Read the model definition and answer for the solid it produces. Units are mm, in the model's axes. A direction names the side the tool comes from. Give positions to 0.01 mm unless a question says otherwise; leave off trailing zeros. Order: outer loops, then holes, each group sorted by start corner. A loop starts at its lowest first (then second) coordinate and runs counter-clockwise, first axis right, second up. Notation, with made-up numbers: M 37.5,21.25 L 60.5,21.25 A18 cw 60.5,51.25 Z; hole C -0.75,-33.75 d10. An arc over 180 degrees is marked long. Write item = value, one per line. Start each with the question number.
from build123d import *
from OCP.BRepFilletAPI import BRepFilletAPI_MakeChamfer

# Parameters (mm, degrees)
CROQUIS1_W              = 175
CROQUIS1_H              = 30
CROQUIS1_W_2            = 16
CROQUIS1_H_2            = 23
SALIENTE_EXTRUIR1_DEPTH = 3
CROQUIS2_W              = 37
CROQUIS2_H              = 30
SALIENTE_EXTRUIR2_DEPTH = 10
CHAFL_N1_SIZE           = 10
CHAFL_N1_SIZE_2         = 8.390996312


with BuildPart() as part:
    # Croquis1 → Saliente-Extruir1 (new body)
    with BuildSketch(Plane(origin=(0, 0, 0), x_dir=(1, 0, 0), z_dir=(0, 1, 0))):
        Rectangle(CROQUIS1_W, CROQUIS1_H)
        with Locations((-75, 0)):
            Rectangle(CROQUIS1_W_2, CROQUIS1_H_2, mode=Mode.SUBTRACT)
        with Locations((30, 0)):
            Rectangle(CROQUIS1_W_2, CROQUIS1_H_2, mode=Mode.SUBTRACT)
        with Locations((-30, 0)):
            Rectangle(CROQUIS1_W_2, CROQUIS1_H_2, mode=Mode.SUBTRACT)
        with Locations((75, 0)):
            Rectangle(CROQUIS1_W_2, CROQUIS1_H_2, mode=Mode.SUBTRACT)
    extrude(amount=SALIENTE_EXTRUIR1_DEPTH)

    # Croquis2 → Saliente-Extruir2 (add)
    with BuildSketch(Plane(origin=(0, 3, 0), x_dir=(1, 0, 0), z_dir=(0, 1, 0))):
        Rectangle(CROQUIS2_W, CROQUIS2_H)
    extrude(amount=SALIENTE_EXTRUIR2_DEPTH)

    # Chaflán1
    chafl_n1_edges_1 = [part.edges().sort_by_distance(p)[0] for p in [
        (18.5, 13, 0),
    ]]
    chafl_n1_side_1 = [part.faces().sort_by_distance(p)[0] for p in [
        (18.5, 12.832180074, 0),
    ]]
    chafl_n1_edges_2 = [part.edges().sort_by_distance(p)[0] for p in [
        (-18.5, 13, 0),
    ]]
    chafl_n1_side_2 = [part.faces().sort_by_distance(p)[0] for p in [
        (-18.5, 12.832180074, 0),
    ]]
    chafl_n1 = BRepFilletAPI_MakeChamfer(part.part.solid().wrapped)
    for e in chafl_n1_edges_1:
        chafl_n1.Add(CHAFL_N1_SIZE - 0.0001, CHAFL_N1_SIZE_2 - 0.0001, e.wrapped, chafl_n1_side_1[0].wrapped)
    for e in chafl_n1_edges_2:
        chafl_n1.Add(CHAFL_N1_SIZE - 0.0001, CHAFL_N1_SIZE_2 - 0.0001, e.wrapped, chafl_n1_side_2[0].wrapped)
    add(Compound.cast(chafl_n1.Shape()), mode=Mode.REPLACE)  # a hair under: the kernel refuses the full size


solid = part.part
1) Each of these flat-tipped pins is pushed along its axis until it touches: P1, Ø1, axis at y = 11, z = 6.5, coming from the +X side; P2, Ø1.5, axis at x = 57, z = 7.5, coming from the +Y side. Where does it stop, or does it pass through?
2) Find section D-D on y = 8.25. Determine the outline of the cut face in (x, z), plus the area to 3 significant figures.
3) Find the intervals of material crossed by probe 1 along X at (y, z) = (0.75, -1); probe 2 along Y at (x, z) = (20.5, 5.5); probe 3 along X at (y, z) = (10, -11.5), in increasing order. Write a range as [from, to].
4) For faces 1 (the face through (-30, 1, 11.5)), 2 (the face through (-14.246, 8.07, 0.21)), 3 (the face through (53, 3, 0)), determine the directions among +Z, -Z, +X, -X, +Y, -Y from which every point of the face is accessible in a straight line to the end or side of a thin tool.
5) Find section C-C on y = 1.5. Determine the outline of the cut face in (x, z).
6) Find section A-A on z = -1.5. Count the separate pieces of the cut face and the enclosed holes in it, plus the area to 3 significant figures.
7) Find section B-B on x = 70.5. Determine the outline of the cut face in (y, z), plus the area to 3 significant figures.
8) For a pull along Z with two mould halves and no side action, classify faces 4 (the face through (75, 1, -11.5)), 5 (the face through (-53, 3, 0)), 6 (the face through (0, 4, 15)) as pulls with the +Z half, pulls with the -Z half, needs draft (parallel to the pull), parting line crosses it, or undercut.
Numbers:
q1.P1 = 12.21
q1.P2 = 3
q2.outline = M -14.09,-15 L 14.09,-15 L 14.09,15 L -14.09,15 Z
q2.area = 846 mm2
q3.probe_1 = [-87.5, -83], [-67, -38], [-22, 22], [38, 67], [83, 87.5]
q3.probe_2 = [0, 3]
q3.probe_3 = [-12.63, 12.63]
q4.face_1 = +Y, -Y
q4.face_2 = +Z, -Z, -X, +Y
q4.face_3 = +Z, -Z, +X, +Y
q5.outline = M -87.5,-15 L 87.5,-15 L 87.5,15 L -87.5,15 Z; hole M -83,-11.5 L -67,-11.5 L -67,11.5 L -83,11.5 Z; hole M -38,-11.5 L -22,-11.5 L -22,11.5 L -38,11.5 Z; hole M 22,-11.5 L 38,-11.5 L 38,11.5 L 22,11.5 Z; hole M 67,-11.5 L 83,-11.5 L 83,11.5 L 67,11.5 Z
q6.separate_pieces = 5
q6.enclosed_holes = 0
q6.area = 619 mm2
q7.outline = M 0,-15 L 3,-15 L 3,-11.5 L 0,-11.5 Z; M 0,11.5 L 3,11.5 L 3,15 L 0,15 Z
q7.area = 21.0 mm2
q8.face_4 = undercut
q8.face_5 = needs draft
q8.face_6 = pulls with the +Z half
